```python
from build123d import *

# Parameters (mm, degrees)
SKETCH_1_W          = 30
SKETCH_1_H          = 750
SKETCH_1_R          = 2.000000003
SKETCH_1_R_2        = 2.000000001
EXTRUDE_2_DEPTH     = 70
SKETCH_2_W          = 26
SKETCH_2_H          = 66
CUT_EXTRUDE_3_DEPTH = 751
CUT_EXTRUDE_4_DEPTH = 71
SKETCH_4_W          = 30
SKETCH_4_H          = 922.920510985
CUT_EXTRUDE_5_DEPTH = 71
SKETCH_5_R          = 3
CUT_EXTRUDE_6_DEPTH = 91


with BuildPart() as part:
    # 草图1 → 凸台-拉伸2 (new body)
    with BuildSketch(Plane.XY):
        Rectangle(SKETCH_1_W, SKETCH_1_H)
        with Locations((-7.5, 363.96878712)):
            Circle(SKETCH_1_R, mode=Mode.SUBTRACT)
        with Locations((7.5, 363.96878712)):
            Circle(SKETCH_1_R, mode=Mode.SUBTRACT)
        with Locations((-7.5, 338.96878712)):
            Circle(SKETCH_1_R, mode=Mode.SUBTRACT)
        with Locations((7.5, 338.96878712)):
            Circle(SKETCH_1_R, mode=Mode.SUBTRACT)
        with Locations((-7.5, -312.867936975)):
            Circle(SKETCH_1_R_2, mode=Mode.SUBTRACT)
        with Locations((7.5, -312.867936975)):
            Circle(SKETCH_1_R_2, mode=Mode.SUBTRACT)
        with Locations((-7.5, -337.867936975)):
            Circle(SKETCH_1_R_2, mode=Mode.SUBTRACT)
        with Locations((7.5, -337.867936975)):
            Circle(SKETCH_1_R_2, mode=Mode.SUBTRACT)
    extrude(amount=EXTRUDE_2_DEPTH)

    # 草图2 → 切除-拉伸3 (cut, through all)
    with BuildSketch(Plane.XZ.offset(375)):
        with Locations((0, 35)):
            Rectangle(SKETCH_2_W, SKETCH_2_H)
    extrude(amount=-CUT_EXTRUDE_3_DEPTH, mode=Mode.SUBTRACT)

    # 草图3 → 切除-拉伸4 (cut, through all)
    with BuildSketch(Plane.XY.offset(70)):
        Polygon((15, -375), (15, -347.1), (-15, -343.150425072), (-15, -375), align=None)
        Polygon((15, 377.040830045), (15, 375), (-15, 371.050425072), (-15, 377.040830045), align=None)
    extrude(amount=-CUT_EXTRUDE_4_DEPTH, mode=Mode.SUBTRACT)

    # 草图4 → 切除-拉伸5 (cut, through all)
    with BuildSketch(Plane(origin=(0, 0, 0), x_dir=(-1, 0, 0), z_dir=(0, 0, -1))):
        with Locations((0, -218.40983042)):
            Rectangle(SKETCH_4_W, SKETCH_4_H)
    extrude(amount=-CUT_EXTRUDE_5_DEPTH, mode=Mode.SUBTRACT)

    # 草图5 → 切除-拉伸6 (cut)
    with BuildSketch(Plane.XY.offset(70)):
        with Locations((-7.5, 363.96878712)):
            Circle(SKETCH_5_R)
        with Locations((7.5, 363.96878712)):
            Circle(SKETCH_5_R)
        with Locations((7.5, 338.96878712)):
            Circle(SKETCH_5_R)
        with Locations((-7.5, 338.96878712)):
            Circle(SKETCH_5_R)
    extrude(amount=-CUT_EXTRUDE_6_DEPTH, mode=Mode.SUBTRACT)


solid = part.part
```
Input: part model. Units: mm. Frame: model coordinates. A direction names the side the tool comes from. Give positions to 0.01 mm unless a question says otherwise; leave off trailing zeros. Order: outer loops, then holes, each group sorted by start corner. A loop starts at its lowest first (then second) coordinate and runs counter-clockwise, first axis right, second up. Notation, with made-up numbers: M 58.5,75 L 116.5,75 A19 cw 116.5,99 Z; hole C -4.5,-30.5 d11. An arc over 180 degrees is marked long. One line per question, with ' | ' between items. Start each with the question number.
1. Section query A-A (z = 41). Return the cut outline in (x, y).
2. Access query for faces 4 (the face through (7.109, 341.943, 1.014)), 5 (the face through (0, 308, 2)). Directions: +Z, -Z, +X, -X, +Y, -Y. A direction counts if a zero-diameter tool reaches every point of the face in a straight line with its end or side. Return the directions, or none.
3. Material intervals for probe 1 along Z at (x, y) = (12, 311.5); probe 2 along X at (y, z) = (364.5, 67); probe 3 along Y at (x, z) = (-7.5, 1.2), sorted ascending. Write a range as [from, to].
4. Pull-direction query (Y, two-part tool) for faces 1 (the face through (7.109, 366.943, 1.014)), 2 (the face through (13.4, 243.05, 32.2)), 3 (the face through (13, 308, 35)); classes: released by +Y, released by -Y, zero draft, split by the parting line, or undercut.
5. Section query C-C (x = -8). Return the cut outline in (y, z).
6. Section query B-B (y = 345). Return the cut outline in (x, z).
7. Section query D-D (x = 2). Return the cut outline in (y, z).
Here are the results:
1) outline: M -15,243.05 L -13,243.05 L -13,371.31 L -15,371.05 Z; M 13,243.05 L 15,243.05 L 15,375 L 13,374.74 Z
2) face 4: +Z, -Z | face 5: +Y, -Y
3) probe 1: [0, 2], [68, 70] | probe 2: [-15, -13], [13, 15] | probe 3: [243.05, 335.97], [341.97, 360.97], [366.97, 372.04]
4) face 1: undercut | face 2: released by -Y | face 3: zero draft
5) outline: M 243.05,0 L 336.01,0 L 336.01,2 L 243.05,2 Z; M 243.05,68 L 336.01,68 L 336.01,70 L 243.05,70 Z; M 341.93,0 L 361.01,0 L 361.01,2 L 341.93,2 Z; M 341.93,68 L 361.01,68 L 361.01,70 L 341.93,70 Z; M 366.93,0 L 371.97,0 L 371.97,2 L 366.93,2 Z; M 366.93,68 L 371.97,68 L 371.97,70 L 366.93,70 Z
6) outline: M -15,0 L 15,0 L 15,70 L -15,70 Z; hole M -13,2 L 13,2 L 13,68 L -13,68 Z
7) outline: M 243.05,0 L 373.29,0 L 373.29,2 L 243.05,2 Z; M 243.05,68 L 373.29,68 L 373.29,70 L 243.05,70 Z
